Geometry: see drawing. Coordinates: mm, zero at the bounding-box minimum. A direction names the side the tool comes from. Give positions to 0.01 mm unless a question says otherwise; leave off trailing zeros. Loops run counter-clockwise (first coordinate to the right, second up) from the corner with the lowest first, then second, coordinate; pieces in that order, holes last. Notation, with made-up numbers: (37, -28) - (74, -28) arc R18 cw to (74, -6) - close; hole circle Ø1 at (65, 62.5). An arc over 180 degrees is marked (long way). Use one line per item in the form item = value.
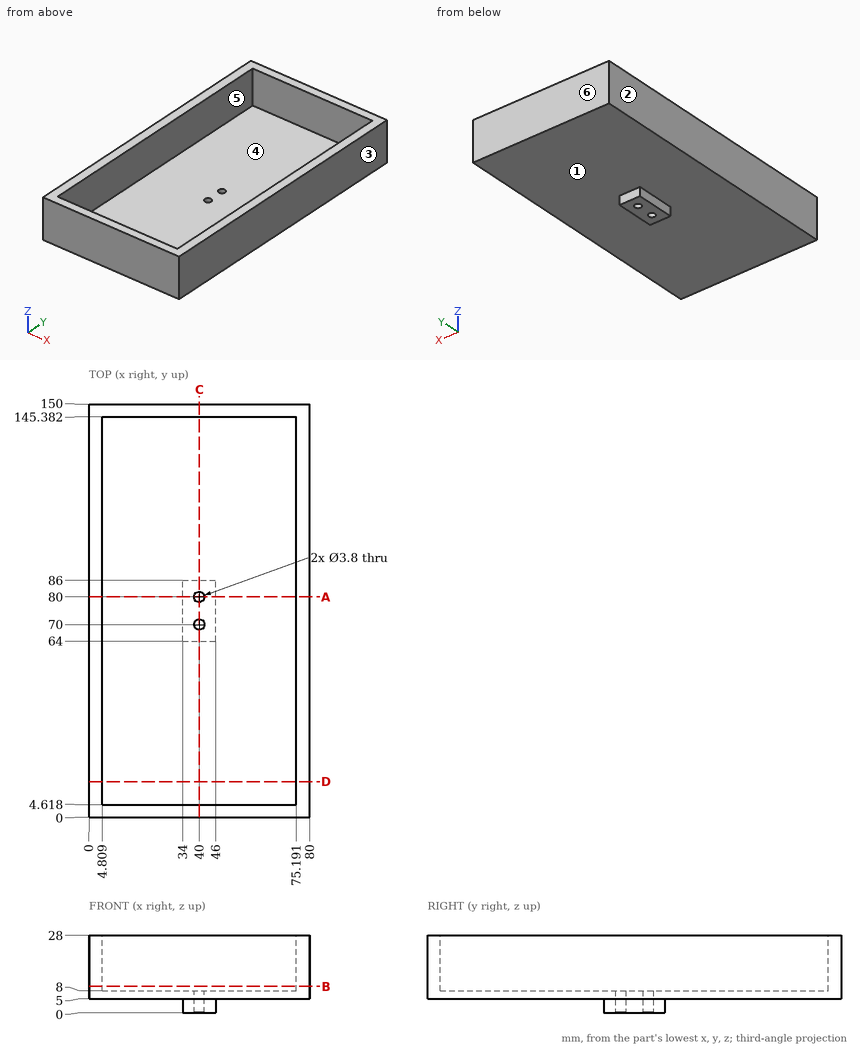
(1) Pull-direction query (X, two-part tool) for the marked faces 1, 2, 3 and 4; classes: released by +X, released by -X, zero draft, split by the parting line, or undercut.
Solution:
face_1 = zero draft
face_2 = released by -X
face_3 = released by +X
face_4 = undercut
(2) Access query for the marked faces 5 and 6. Directions: +Z, -Z, +X, -X, +Y, -Y. A direction counts if a zero-diameter tool reaches every point of the face in a straight line with its end or side. Return the directions, or none.
Solution:
face_5 = +Z
face_6 = +Z, -Z, +X, -X, +Y
(3) Pin query (flat end, axial travel): P1, Ø6, axis at x = 36.5, y = 32.5, coming from the -Z side; P2, Ø6, axis at x = 40, y = 80, coming from the +Z side; P3, Ø1.5, axis at y = 74, z = 1.5, coming from the -X side. Return the tip coordinate at first contact, or that it passes through.
Solution:
P1 = 5
P2 = 8
P3 = 34
(4) Material intervals for L1, parallel to X at y = 80, z = 5.75; L2, parallel to Y at x = 26, z = 12.5; L3, parallel to X at y = 80, z = 4.75, sorted ascending. Write a range as from..to.
Solution:
L1 = 0..38.1, 41.9..80
L2 = 0..4.62, 145.38..150
L3 = 34..38.1, 41.9..46
(5) Cut plane D-D (y = 13). Return the cut outline in (x, z).
Solution:
outline = (0, 5) - (80, 5) - (80, 28) - (75.19, 28) - (75.19, 8) - (4.81, 8) - (4.81, 28) - (0, 28) - close
(6) Cut plane C-C (x = 40). Return the cut outline in (y, z), plus the area to 3 significant figures.
Solution:
outline = (0, 5) - (64, 5) - (64, 0) - (68.1, 0) - (68.1, 8) - (4.62, 8) - (4.62, 28) - (0, 28) - close; (71.9, 0) - (78.1, 0) - (78.1, 8) - (71.9, 8) - close; (81.9, 0) - (86, 0) - (86, 5) - (150, 5) - (150, 28) - (145.38, 28) - (145.38, 8) - (81.9, 8) - close
area = 684 mm2
(7) Cut plane A-A (y = 80). Return the cut outline in (x, z).
Solution:
outline = (0, 5) - (34, 5) - (34, 0) - (38.1, 0) - (38.1, 8) - (4.81, 8) - (4.81, 28) - (0, 28) - close; (41.9, 0) - (46, 0) - (46, 5) - (80, 5) - (80, 28) - (75.19, 28) - (75.19, 8) - (41.9, 8) - close
(8) Cut plane B-B (z = 9.5). Return the cut outline in (x, y).
Solution:
outline = (0, 0) - (80, 0) - (80, 150) - (0, 150) - close; hole (4.81, 4.62) - (75.19, 4.62) - (75.19, 145.38) - (4.81, 145.38) - close
